Could you check a few things on this model? Use its own coordinates, in mm. A direction names the side the tool comes from. Coordinates: 2 decimals unless noted, no trailing zeros. Loops run counter-clockwise (first coordinate to the right, second up) from the corner with the lowest first, then second, coordinate; pieces in that order, holes last. Notation, with made-up numbers: M 4.25,76 L 38.25,76 A19 ccw 38.25,80 Z; hole C 48.25,52.25 d6. An arc over 180 degrees is marked long. Use one line per item in the form item = value. Start each with the question number.
```python
from build123d import *

# Parameters (mm, degrees)
SKETCH1_W           = 80
SKETCH1_H           = 50
BOSS_EXTRUDE1_DEPTH = 3.175
SKETCH2_W           = 5
SKETCH2_H           = 3.175
BOSS_EXTRUDE2_DEPTH = 2.5
LPATTERN1_COUNT     = 5
LPATTERN1_PITCH     = 10
SKETCH3_W           = 5
SKETCH3_H           = 3.175
BOSS_EXTRUDE3_DEPTH = 2.5
LPATTERN2_COUNT     = 5
LPATTERN2_PITCH     = 10
SKETCH4_W           = 5
SKETCH4_H           = 3.175
BOSS_EXTRUDE4_DEPTH = 2.5
LPATTERN3_COUNT     = 8
LPATTERN3_PITCH     = 10


with BuildPart() as part:
    # Sketch1 → Boss-Extrude1 (new body)
    with BuildSketch(Plane(origin=(0, 0, 0), x_dir=(1, 0, 0), z_dir=(0, 1, 0))):
        with Locations((40, 25)):
            Rectangle(SKETCH1_W, SKETCH1_H)
    extrude(amount=BOSS_EXTRUDE1_DEPTH)

    # Sketch2 → Boss-Extrude2 (add)
    with BuildSketch(Plane.ZY):
        with Locations((-2.5, 1.5875)):
            Rectangle(SKETCH2_W, SKETCH2_H)
    boss_extrude2 = extrude(amount=BOSS_EXTRUDE2_DEPTH)

    # LPattern1: Boss-Extrude2 ×5
    with Locations(*[(0, 0, -i * LPATTERN1_PITCH) for i in range(1, LPATTERN1_COUNT)]):
        add(boss_extrude2)

    # Sketch3 → Boss-Extrude3 (add)
    with BuildSketch(Plane(origin=(80, 0, 0), x_dir=(0, 0, -1), z_dir=(1, 0, 0))):
        with Locations((2.5, 1.5875)):
            Rectangle(SKETCH3_W, SKETCH3_H)
    boss_extrude3 = extrude(amount=BOSS_EXTRUDE3_DEPTH)

    # LPattern2: Boss-Extrude3 ×5
    with Locations(*[(0, 0, -i * LPATTERN2_PITCH) for i in range(1, LPATTERN2_COUNT)]):
        add(boss_extrude3)

    # Sketch4 → Boss-Extrude4 (add)
    with BuildSketch(Plane.XY):
        with Locations((77.5, 1.5875)):
            Rectangle(SKETCH4_W, SKETCH4_H)
    boss_extrude4 = extrude(amount=BOSS_EXTRUDE4_DEPTH)

    # LPattern3: Boss-Extrude4 ×8
    with Locations(*[(-i * LPATTERN3_PITCH, 0, 0) for i in range(1, LPATTERN3_COUNT)]):
        add(boss_extrude4)


solid = part.part
```
Item 1: Please list where these lines run through material, in increasing order: line 1 along Z through (x, y) = (14.5, 0.45); line 2 along X through (y, z) = (0.3, -9).
Item 2: I want a section at A-A (z = -28.5). Write out the boundary of the cut face in (x, y) (3 decimals), plus the area to 3 significant figures.
Item 3: Thinking about a two-plate mould opening in Z: for faces 6 (the flat face through (-1, 2, -20)), 7 (the flat face through (82.5, 2, -42)), 8 (the flat face through (52, 2, 0)), which applies, pulls with the +Z half, pulls with the -Z half, needs draft (parallel to the pull), parting line crosses it, or undercut?
Item 4: For faces 1 (the flat face through (50, 2, 1)), 2 (the flat face through (81, 2, -15)), 3 (the flat face through (0, 2, -17)), 4 (the flat face through (0, 2, -47)), 5 (the flat face through (5, 2, 1)), which set-ups out of +Z, -Z, +X, -X, +Y, -Y let a thin tool reach every point of the face, with its end or its side?
Item 5: I'm going to push flat-ended pins straight in: P1, Ø1.2, axis at y = 1.5, z = 1, coming from the -X side; P2, Ø1.2, axis at y = 1, z = 0.5, coming from the -X side; P3, Ø1.5, axis at y = 1, z = -27.5, coming from the +X side; P4, Ø1, axis at y = 2, z = -8.5, coming from the -X side. Where does each tip first touch, or does it pass through?
Worked answers:
q1.line_1 = -50 to 0
q1.line_2 = 0 to 80
q2.outline = M 0,0 L 80,0 L 80,3.175 L 0,3.175 Z
q2.area = 254 mm²
q3.face_6 = undercut
q3.face_7 = needs draft
q3.face_8 = pulls with the +Z half
q4.face_1 = +Z, +Y, -Y
q4.face_2 = +X, +Y, -Y
q4.face_3 = -X, +Y, -Y
q4.face_4 = -Z, -X, +Y, -Y
q4.face_5 = +Z, -X, +Y, -Y
q5.P1 = 5
q5.P2 = -2.5
q5.P3 = 80
q5.P4 = 0
